```python
from build123d import *

# Parameters (mm, degrees)
F1_W          = 50.8
F1_H          = 38.1
F2_DEPTH      = 6.985
F4_DEPTH      = 50.8
F6_DEPTH      = 15.24
F6_DEPTH_BACK = 15.24
F7_W          = 20
F7_H          = 15.8292923384
F8_DEPTH      = 25.4
F9_R          = 1.6
F10_DEPTH     = 25.4
F11_R         = 1.6
F12_DEPTH     = 5.7
F13_W         = 30.48
F13_H         = 2
F14_DEPTH     = 2
F14_TAPER     = 10
F15_R         = 0.508
F16_R         = 5.08
F17_R         = 1.27


# Not quite as in the source:
# - two fillets or chamfers of one size are made in one step


with BuildPart() as f2:
    # F1 (on Top) → F2 (new body)
    with BuildSketch(Plane.XY):
        Rectangle(F1_W, F1_H)
    extrude(amount=-F2_DEPTH)

    # F3 (on face) → F4 (cut, through all)
    with BuildSketch(Plane.YZ.offset(25.4)):
        with BuildLine():
            add(Edge.make_bspline(
                [(-4.125, 4.125), (-2.4255892558, 4.1137489608), (-0.0276085061, 2.971292738), (2.5249406681, 4.1137612248), (4.191, 4.191)],
                knots=[0, 0, 0, 0, 0.4977710734, 1, 1, 1, 1], degree=3))
            ThreePointArc((-4.125, 4.125), (-7.0418154724, 2.9168154724), (-8.25, 0))
            ThreePointArc((-8.25, 0), (-7.0418154724, -2.9168154724), (-4.125, -4.125))
            add(Edge.make_bspline(
                [(-4.125, -4.125), (-2.9335741419, -4.2006121948), (0.4172014685, -3.0581585459), (2.1438994445, -4.2006121948), (4.191, -4.191)],
                knots=[0, 0, 0, 0, 0.497799261, 1, 1, 1, 1], degree=3))
            ThreePointArc((4.191, -4.191), (7.15448452, -2.96348452), (8.382, 0))
            ThreePointArc((8.382, 0), (7.15448452, 2.96348452), (4.191, 4.191))
        make_face()
    extrude(amount=-F4_DEPTH, mode=Mode.SUBTRACT)

    # F5 (on Right) → F6 (join, two sides)
    with BuildSketch(Plane.YZ) as f6_sk:
        with BuildLine():
            ThreePointArc((-32.258, -38.6095089919), (0, -24.985), (32.258, -38.6095089919))
            Line((32.258, -38.6095089919), (31.75, -34.0955424944))
            ThreePointArc((31.75, -34.0955424944), (22.9296157026, -27.265073299), (12.7, -22.8142923384))
            ThreePointArc((12.7, -22.8142923384), (0, -20.985), (-12.7, -22.8142923384))
            ThreePointArc((-12.7, -22.8142923384), (-22.9296157026, -27.265073299), (-31.75, -34.0955424944))
            Line((-31.75, -34.0955424944), (-32.258, -38.6095089919))
        make_face()
        with BuildLine():
            ThreePointArc((-12.7, -22.8142923384), (0, -20.985), (12.7, -22.8142923384))
            Line((12.7, -22.8142923384), (12.7, -6.985))
            Line((12.7, -6.985), (-12.7, -6.985))
            Line((-12.7, -6.985), (-12.7, -22.8142923384))
        make_face()
    extrude(amount=F6_DEPTH)
    extrude(f6_sk.sketch, amount=-F6_DEPTH_BACK)

    # F7 (on face) → F8 (cut)
    with BuildSketch(Plane.XZ.offset(12.7)):
        with Locations((0, -14.8996461692)):
            Rectangle(F7_W, F7_H)
    extrude(amount=-F8_DEPTH, mode=Mode.SUBTRACT)

    # F9 (on face) → F10 (cut)
    with BuildSketch(Plane(origin=(0, 0, -6.985), x_dir=(1, 0, 0), z_dir=(0, 0, -1))):
        with Locations((20.32, -13.97)):
            Circle(F9_R)
        with Locations((-20.32, -13.97)):
            Circle(F9_R)
        with Locations((-20.32, 13.97)):
            Circle(F9_R)
        with Locations((20.32, 13.97)):
            Circle(F9_R)
    extrude(amount=-F10_DEPTH, mode=Mode.SUBTRACT)

    # F11 (on face) → F12 (cut)
    with BuildSketch(Plane(origin=(0, 0, -6.985), x_dir=(1, 0, 0), z_dir=(0, 0, -1))):
        Polygon((21.645, -16.26496732), (22.97, -13.97), (21.645, -11.67503268), (18.995, -11.67503268), (17.67, -13.97), (18.995, -16.26496732), align=None)
        with Locations((20.32, -13.97)):
            Circle(F11_R, mode=Mode.SUBTRACT)
        Polygon((-18.995, -11.67503268), (-21.645, -11.67503268), (-22.97, -13.97), (-21.645, -16.26496732), (-18.995, -16.26496732), (-17.67, -13.97), align=None)
        with Locations((-20.32, -13.97)):
            Circle(F11_R, mode=Mode.SUBTRACT)
        Polygon((-18.995, 11.67503268), (-17.67, 13.97), (-18.995, 16.26496732), (-21.645, 16.26496732), (-22.97, 13.97), (-21.645, 11.67503268), align=None)
        with Locations((-20.32, 13.97)):
            Circle(F11_R, mode=Mode.SUBTRACT)
        Polygon((18.995, 11.67503268), (21.645, 11.67503268), (22.97, 13.97), (21.645, 16.26496732), (18.995, 16.26496732), (17.67, 13.97), align=None)
        with Locations((20.32, 13.97)):
            Circle(F11_R, mode=Mode.SUBTRACT)
    extrude(amount=-F12_DEPTH, mode=Mode.SUBTRACT)

    # F13 (on face) → F14 (join)
    with BuildSketch(Plane.XY):
        with Locations((0, 14.24)):
            Rectangle(F13_W, F13_H)
        with Locations((0, -14.24)):
            Rectangle(F13_W, F13_H)
    extrude(amount=F14_DEPTH, taper=F14_TAPER)

    # F15
    f15_edges = [f2.edges().sort_by_distance(p)[0] for p in [
        (0, 32.258, -38.609509),
        (0, -32.258, -38.609509),
    ]]
    fillet(f15_edges, radius=F15_R)

    # F16
    f16_edges = [f2.edges().sort_by_distance(p)[0] for p in [
        (0, 31.75, -34.095542),
        (0, -31.75, -34.095542),
    ]]
    fillet(f16_edges, radius=F16_R)

    # F17
    f17_edges = [f2.edges().sort_by_distance(p)[0] for p in [
        (-15.24, 0, -6.985),
        (12.62, -12.7, -22.814292),
        (-12.62, -12.7, -22.814292),
        (-12.62, -12.7, -6.985),
        (0, 19.05, -6.985),
        (25.4, 0, -6.985),
        (-25.4, 0, -6.985),
        (0, -19.05, -6.985),
        (-12.62, 12.7, -6.985),
        (-10, 0, -6.985),
        (12.62, -12.7, -6.985),
        (10, 0, -6.985),
        (15.24, 0, -6.985),
        (12.62, 12.7, -6.985),
        (-12.62, 12.7, -22.814292),
        (12.62, 12.7, -22.814292),
        (25.4, 19.05, -3.4925),
        (-25.4, 19.05, -3.4925),
        (25.4, -19.05, -3.4925),
        (-25.4, -19.05, -3.4925),
    ]]
    fillet(f17_edges, radius=F17_R)


solid = f2.part
```
Design review of the part built by this model. Coordinates are the model's own, in mm. A direction names the side the tool comes from. Coordinates: 2 decimals unless noted, no trailing zeros. Loops run counter-clockwise (first coordinate to the right, second up) from the corner with the lowest first, then second, coordinate; pieces in that order, holes last.
Q1. Tool access review of faces 4 (the face through (13, -12.7, -15)), 5 (the face through (-20, -16.265, -4)), 6 (the face through (-15.24, 0, -22)): name each direction out of +Z, -Z, +X, -X, +Y, -Y from which nothing blocks a thin tool from reaching the whole face with its end or side.
Reported:
face 4: +X, -X, -Y
face 5: -Z
face 6: -Z, -X, +Y, -Y
Q2. The part is to be moulded in two halves that separate along Z. For faces 1 (the face through (0, 19.05, -3)), 2 (the face through (0, -12, 0)), 3 (the face through (-13, -12.7, -15)), say which applies: +Z half, -Z half, draft (parallel to the pull), parting line (faces both ways), or undercut.
Reported:
face 1: draft
face 2: +Z half
face 3: undercut
Q3. We need section D-D on y = 22. State the section outline as (x, z) points.
Reported:
outline: (-15.24, -30.73) - (15.24, -30.73) - (15.24, -26.73) - (-15.24, -26.73) - close
Q4. To check wall thickness, follow line 1 (X direction, y = -13.97, z = -0.6); line 2 (Y direction, x = 20.32, z = -0.3); line 3 (X direction, y = -13, z = -1). State the ranges of each line that lie inside material, in increasing order.
Reported:
line 1: x = -25.4 to -21.92, -18.72 to 18.72, 21.92 to 25.4
line 2: y = -19.05 to -15.57, -12.37 to -8.24, 8.37 to 12.37, 15.57 to 19.05
line 3: x = -25.4 to -21.59, -19.05 to 19.05, 21.59 to 25.4
Q5. We need section A-A on z = -27. State the section outline as (x, y) points.
Reported:
outline: (-15.24, -22.48) - (15.24, -22.48) - (15.24, -13.32) - (-15.24, -13.32) - close; (-15.24, 13.32) - (15.24, 13.32) - (15.24, 22.48) - (-15.24, 22.48) - close
Q6. We need section C-C on x = -20.32. State how many separate pieces and enclosed holes the cut face has, and give its area (3 significant figures).
Reported:
separate pieces: 3
enclosed holes: 0
area: 145 mm2
Q7. For pin 1 (2 mm diameter, centred on x = 20, z = -4, fed in from -Y); pin 2 (10 mm diameter, centred on x = 0, y = 0, fed in from +Z); pin 3 (3 mm diameter, centred on x = 16, z = -21, fed in from +Y); pin 4 (2.5 mm diameter, centred on x = -20.32, y = -13.97, fed in from -Z), all flat-tipped, find the tip position at first contact; note any pin that passes through.
Reported:
pin 1: stops at y = -19.05
pin 2: stops at z = -3.63
pin 3: stops at y = 12.77
pin 4: passes through
Q8. We need section B-B on y = -5. State the section outline as (x, z) points (3 decimals).
Reported:
outline: (-25.4, -5.715) arc R1.27 ccw to (-24.13, -6.985) - (-16.51, -6.985) arc R1.27 cw to (-15.24, -8.255) - (-15.24, -25.264) - (15.24, -25.264) - (15.24, -8.255) arc R1.27 cw to (16.51, -6.985) - (24.13, -6.985) arc R1.27 ccw to (25.4, -5.715) - (25.4, -4.031) - (-25.4, -4.031) - close; hole (-10, -22.814) - (10, -22.814) - (10, -8.255) arc R1.27 ccw to (8.73, -6.985) - (-8.73, -6.985) arc R1.27 ccw to (-10, -8.255) - close
